Model file for the job. Use its own axes, mm. Face numbers are marked on the shaded views. A direction names the side the tool comes from. Round coordinates to 2 decimals unless told otherwise and drop trailing zeros. Order: outer loops, then holes, each group sorted by start corner. A loop starts at its lowest first (then second) coordinate and runs counter-clockwise, first axis right, second up. Notation, with made-up numbers: (85, 27.5) - (138, 27.5) arc R12 cw to (138, 50.5) - close; hole circle Ø1 at (-37, 79.25). An arc over 180 degrees is marked (long way). Use one line per item in the form item = value.
from build123d import *

# Parameters (mm, degrees)
SKETCH1_R           = 3.1496
BOSS_EXTRUDE1_DEPTH = 13.208
SKETCH2_R           = 6.35
BOSS_EXTRUDE2_DEPTH = 7.8867
BOSS_EXTRUDE3_DEPTH = 11.7094
SKETCH4_R           = 5.0292
BOSS_EXTRUDE4_DEPTH = 1.1684
BOSS_EXTRUDE5_DEPTH = 143.51


with BuildPart() as part:
    # Sketch1 → Boss-Extrude1 (new body)
    with BuildSketch(Plane(origin=(0, 0, 0), x_dir=(1, 0, 0), z_dir=(0, 1, 0))):
        Circle(SKETCH1_R)
    extrude(amount=BOSS_EXTRUDE1_DEPTH)

    # Sketch2 → Boss-Extrude2 (add)
    with BuildSketch(Plane(origin=(0, 13.208, 0), x_dir=(1, 0, 0), z_dir=(0, 1, 0))):
        Circle(SKETCH2_R)
    extrude(amount=BOSS_EXTRUDE2_DEPTH)

    # Sketch3 → Boss-Extrude3 (add)
    with BuildSketch(Plane(origin=(0, 21.0947, 0), x_dir=(1, 0, 0), z_dir=(0, 1, 0))):
        Polygon((3.828614027, -6.253402911), (7.329912794, 0.188975553), (3.501298767, 6.442378464), (-3.828614027, 6.253402911), (-7.329912794, -0.188975553), (-3.501298767, -6.442378464), align=None)
    extrude(amount=BOSS_EXTRUDE3_DEPTH)

    # Sketch4 → Boss-Extrude4 (add)
    with BuildSketch(Plane(origin=(0, 32.8041, 0), x_dir=(1, 0, 0), z_dir=(0, 1, 0))):
        Circle(SKETCH4_R)
    extrude(amount=BOSS_EXTRUDE4_DEPTH)

    # Sketch5 → Boss-Extrude5 (add)
    with BuildSketch(Plane(origin=(0, 33.9725, 0), x_dir=(1, 0, 0), z_dir=(0, 1, 0))):
        Polygon((-3.828614027, 6.253402911), (-7.329912794, -0.188975553), (-3.501298767, -6.442378464), (3.828614027, -6.253402911), (7.329912794, 0.188975553), (3.501298767, 6.442378464), align=None)
    extrude(amount=BOSS_EXTRUDE5_DEPTH)


solid = part.part
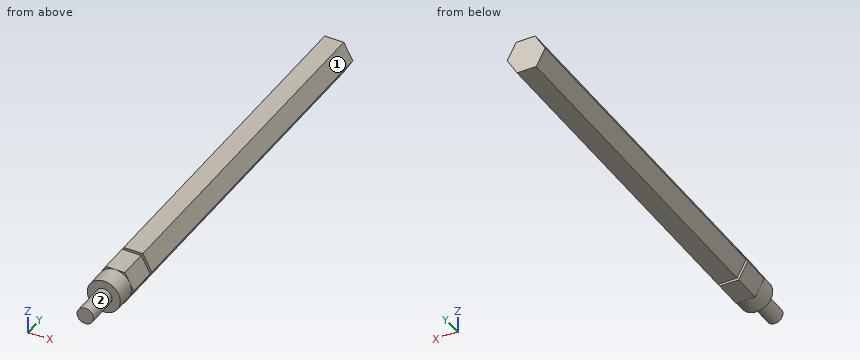
(1) Pin check, flat tips, straight feed: pin 1 (0.9 mm diameter, centred on x = -2, z = 4.5, fed in from -Y); pin 2 (2 mm diameter, centred on y = 77, z = -1.5, fed in from -X); pin 3 (1 mm diameter, centred on y = 45.5, z = 2.5, fed in from -X). Stop position of each tip, or through.
Report:
pin_1 = 13.21
pin_2 = -6.96
pin_3 = -6.22
(2) Slice it at A-A on y = 98. Give the cut face in (x, z).
Report:
outline = (-7.33, 0.19) - (-3.83, -6.25) - (3.5, -6.44) - (7.33, -0.19) - (3.83, 6.25) - (-3.5, 6.44) - close
(3) Probe probe 1 along Y at (x, z) = (-2, -5.25); probe 2 along X at (y, z) = (15, -0.25); probe 3 along Y at (x, z) = (-3.25, 5.5). List the from-to ranges inside material, lowest first. Write a range as [from, to].
Report:
probe_1 = [13.21, 32.8], [33.97, 177.48]
probe_2 = [-6.35, 6.35]
probe_3 = [21.09, 32.8], [33.97, 177.48]
(4) Tool access for the marked faces 1 and 2: list every direction of +Z, -Z, +X, -X, +Y, -Y with a clear straight run to the whole face (end or side of a thin tool).
Report:
face_1 = +Z, +X, +Y, -Y
face_2 = -Y
